Design review of the part built by this model. Coordinates are the model's own, in mm. Coordinates: 2 decimals unless noted, no trailing zeros. Loops run counter-clockwise (first coordinate to the right, second up) from the corner with the lowest first, then second, coordinate; pieces in that order, holes last. Notation, with made-up numbers: (-36, 74.25) - (-16, 74.25) arc R16 ccw to (-16, 103.25) - close; hole circle Ø11 at (5.5, 49.5). An arc over 180 degrees is marked (long way). Use one line per item in the form item = value. Start each with the question number.
(1) Add section A-A (x = 50.8). State the section outline as (y, z) points, plus the area to 3 significant figures.
(2) For L1, parallel to X at y = 57, z = 2.8; L2, parallel to X at y = 13, z = 4.8; L3, parallel to X at y = 53.5, z = 2.7, list the stretches that pass through material, from the lowest coordinate up.
(3) Clearance check with a flat-ended pin moving along its axis: pin 1 Ø1 at (x, y) = (276.5, 53) entering from -Z. State where the tip first meets the part, or that it passes through.
(4) Add section B-B (z = 4.3). Count the separate pieces of the cut face and the enclosed holes in it, plus the area to 3 significant figures.
Autodesk Inventor part; units mm, degrees
ref_plane "YZ Plane" through (0, 0, 0) normal (1, 0, 0) x (0, 1, 0)
ref_plane "XZ Plane" through (0, 0, 0) normal (0, 1, 0) x (-1, 0, 0)
ref_plane "XY Plane" through (0, 0, 0) normal (0, 0, 1) x (1, 0, 0)
sketch "Sketch1" plane through (0, 0, 0) normal (0, 0, 1) x (1, 0, 0)
  line L0 (0, 121.6177) -> (0, -51.755)
  line L1 (-63.9166, 0) -> (383.4994, 0)
  line L2 (0, 0) -> (319.5828, 0)
  line L3 (319.5828, 0) -> (319.5828, 69.85)
  line L4 (319.5828, 69.85) -> (0, 69.85)
  line L5 (0, 69.85) -> (0, 0)
  line L6 (9.525, 14.2875) -> (92.075, 14.2875) construction
  circle A0 centre (50.8, 14.2875) radius 41.275 construction
  line L7 (0, 34.925) -> (319.5828, 34.925) construction
  circle A1 centre (266.7, 77.8002) radius 19.05
  circle A2 centre (127, 1.6002) radius 7.62
  point P0 (50.8, 55.5625)
  point P1 (310.4515, 57.15)
  point P2 (310.4515, 12.7)
  dimension "d0" = 319.5828
  dimension "d1" = 69.85
  dimension "d2" = 82.55
  dimension "d5" = 14.2875
  dimension "d7" = 14.2875
  dimension "d8" = 9.525
  dimension "d9" = 9.1313
  dimension "d10" = 22.225
  dimension "d11" = 22.225
  dimension "d29" = 266.7
  dimension "d30" = 7.9502
  dimension "d31" = 38.1
  dimension "d35" = 15.24
  dimension "d36" = 1.6002
  dimension "d37" = 127
extrude "Extrusion1" add sketch "Sketch1" along normal blind 5.842 contours L4 A1 L3 L1 A2 L0 | L4 A1 | A2 L1 picked at (261.678, 68.614) picked at (126.7265, 4.018)
hole "Hole1" at (310.4515, 57.15, 0) at (310.4515, 12.7, 0) direction (0, 0, 1) diameter 3.81 end through all
hole "Hole2" at (9.525, 14.2875, 0) at (92.075, 14.2875, 0) at (50.8, 55.5625, 0) direction (0, 0, 1) diameter 5.588 end through all
fillet "Fillet1" radius 6.35 2 edges at (0, 69.85, 2.921) (0, 0, 2.921)
extrude "Extrusion2" cut sketch "Sketch1" along normal up to next contours A1 L4 | L4 A1 | A2 L1 | L1 A2
fillet "Fillet2" radius 3.175 4 edges at (249.3882, 69.85, 2.921) (284.0118, 69.85, 2.921) (134.4501, 0, 2.921) (119.5499, 0, 2.921)
sketch "Sketch2" plane through (0, 0, 5.842) normal (0, 0, 1) x (1, 0, 0)
  point P0 (0, 0)
equation "\"d5\" = d7"
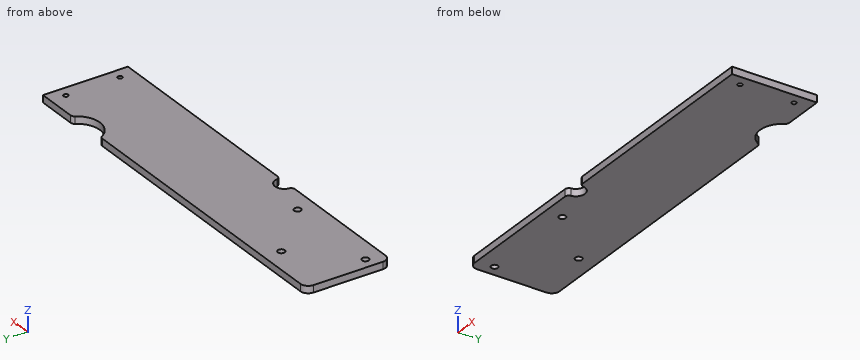
Computed values:
q1.outline = (0, 0) - (52.77, 0) - (52.77, 5.84) - (0, 5.84) - close; (58.36, 0) - (69.85, 0) - (69.85, 5.84) - (58.36, 5.84) - close
q1.area = 375 mm^2
q2.L1 = 0 to 48.4, 53.2 to 308.55, 312.35 to 319.58
q2.L2 = 0 to 7.05, 12 to 89.6, 94.55 to 308.57, 312.33 to 319.58
q2.L3 = 0 to 48.92, 52.68 to 319.58
q3.pin_1 = 0
q4.separate_pieces = 1
q4.enclosed_holes = 5
q4.area = 21,800 mm^2
